Solid Edge part; units mm, degrees
sketch "Sketch1" plane through (0, 0, 0) normal (1, 0, 0) x (0, 1, 0)
  circle A0 centre (0, 0) radius 32
  circle A1 centre (0, 0) radius 16
extrude "Protrusion1" add sketch "Sketch1" against normal blind 70
sketch "Sketch2" plane through (0, 0, 0) normal (0, -1, 0) x (1, 0, 0)
  line L0 (-70, 32) -> (-36.8752, 123.9402)
  line L1 (0, 32) -> (0, 117.5)
  line L2 (0, 19.9591) -> (0, 32)
  line L3 (-70, 19.9591) -> (0, 19.9591)
  line L4 (-70, 32) -> (-70, 19.9591)
  arc A0 (-36.8752, 123.9402) -> (0, 117.5) centre (-19, 117.5) cw
extrude "ExtrudedProtrusion_6" add sketch "Sketch2" along normal mid plane 16
pattern_circular "Pattern1" count 3 over 360 about axis through (-70, 0, 0) along (-1, 0, 0) of "ExtrudedProtrusion_6"
sketch "Sketch3" plane through (0, 0, 25.9109) normal (1, 0, 0) x (0, -0.866, 0.5)
  line L0 (-29.1919, 50.0144) -> (-63.936, 110.2076)
  line L1 (-44.9554, 22.4395) -> (-114.4554, 22.4395)
  arc A0 (-114.4554, 22.4395) -> (-63.936, 110.2076) centre (-12.9554, 22.4395) cw
  arc A1 (-44.9554, 22.4395) -> (-29.1919, 50.0144) centre (-12.9554, 22.4395) cw
  circle A2 centre (-87.5005, 65.3234) radius 8
extrude "ExtrudedProtrusion_7" add sketch "Sketch3" against normal blind 19
pattern_circular "Pattern3" count 6 over 360 about axis through (0, 0, 0) along (-1, 0, 0) of "ExtrudedProtrusion_7"
sketch "Sketch4" plane through (-35, 76.5226, -34.9428) normal (0, 0.5, 0.866) x (0, 0.866, -0.5)
  circle A0 centre (33.7581, -16) radius 8
extrude "ExtrudedCutout_3" cut sketch "Sketch4" against normal blind 16
pattern_circular "Pattern4" count 3 over 360 about axis through (0, 0, 0) along (-1, 0, 0) of "ExtrudedCutout_3"
CAD build for the part. Positions are in the model's coordinates, mm. A direction names the side the tool comes from. Coordinates: 2 decimals unless noted, no trailing zeros. Order: outer loops, then holes, each group sorted by start corner. A loop starts at its lowest first (then second) coordinate and runs counter-clockwise, first axis right, second up. Notation, with made-up numbers: (-28.5, 24) - (10.5, 24) arc R17 cw to (10.5, 45) - close; hole circle Ø1 at (80, 12.25). An arc over 180 degrees is marked (long way). Use a Markdown table: item, result. Add a question column.
(1) Saw through at A-A (y = -55). Give the cut face in (x, z), then the cut area to 3 significant figures.
(2) Saw through at B-B (x = -54.5). Give the cut face in (y, z), then the cut area to 3 significant figures.
(3) Saw through at D-D (z = 0). Give the cut face in (x, y).
(4) Saw through at C-C (z = -36). Give the cut face in (x, y).
(5) Drill centre lines: line 1 along Y through (x, z) = (-14.5, 69); line 2 along Z through (x, y) = (-13.5, 79.5); line 3 along Y through (x, z) = (-32.5, -72). Where is each one in solid material? Low to high. Write a range as [from, to].
(6) Which spindle directions (+Z, -Z, +X, -X, +Y, -Y) get a long thin tool onto all of the face, cutting with end or side? Do faces 1 (the face through (-19, 38, 59)), 2 (the face through (-34.51, -57.73, -42.57)), 3 (the face through (-9.367, -57.52, 32.897)). Say none if no direction does.
(7) Pull direction Y, two halves, no side cores. Call faces 4 (the face through (-9.367, -57.386, 33.132)), 5 (the face through (0, -1, -18)), 6 (the face through (-53.67, 66.91, -38.76)), 7 (the face through (-9.367, -101.398, 4.556)): +Y half, -Y half, draft (parallel to the pull), parting line (faces both ways), or undercut.
(8) Flat gauge pins, fed straight in: pin 1 (3 mm diameter, centred on x = -15, z = 5, fed in from -Y); pin 2 (10 mm diameter, centred on x = -41, z = -24.5, fed in from +Y); pin 3 (9.5 mm diameter, centred on x = -12, z = -74, fed in from +Y); pin 4 (13 mm diameter, centred on y = 86, z = 0.13, fed in from -X). Where does each tip first touch, or does it go through?
Solved:
| question | item | result |
|---|---|---|
| 1 | outline | (-60.31, -22.52) - (-56.98, -40.99) - (-19, -40.99) - (-19, -85.31) - (0, -85.31) - (0, 31.44) - (-19, 31.44) - (-19, -22.52) - close; (-19, 31.75) - (0, 31.75) - (0, 85.31) - (-19, 85.31) - close |
| 1 | area | 3,970 mm² |
| 2 | outline | (-68.97, -30.58) - (-60.97, -44.44) - (-22.83, -22.42) arc R32 ccw to (22.83, -22.42) - (60.97, -44.44) - (68.97, -30.58) - (30.83, -8.56) arc R32 ccw to (8, 30.98) - (8, 75.02) - (-8, 75.02) - (-8, 30.98) arc R32 ccw to (-30.83, -8.56) - close; hole circle Ø32 at (0, 0) |
| 2 | area | 4,490 mm² |
| 3 | outline | (-70, -32) - (-19, -32) - (-19, -78) - (0, -78) - (0, -16) - (-70, -16) - close; (-70, 16) - (0, 16) - (0, 78) - (-19, 78) - (-19, 32) - (-70, 32) - close; (-19, -101.5) - (0, -101.5) - (0, -94) - (-19, -94) - close; (-19, 94) - (0, 94) - (0, 101.5) - (-19, 101.5) - close |
| 4 | outline | (-60.58, -46.35) - (-50.6, -78.35) - (-19, -78.35) - (-19, -94.9) - (0, -94.9) - (0, 0) - (-19, 0) - (-19, -46.35) - close; (-60.58, 46.35) - (-19, 46.35) - (-19, 0.27) - (0, 0.27) - (0, 94.9) - (-19, 94.9) - (-19, 78.35) - (-50.6, 78.35) - close |
| 5 | line 1 | y = [-74.44, -49.01], [-37.22, 37.12], [48.65, 74.44] |
| 5 | line 2 | z = [-63.1, -4.53], [4.8, 45.9], [46.21, 63.1] |
| 5 | line 3 | y = [-109.55, -108.71], [108.71, 109.55] |
| 6 | face 1 | +Z, -X, +Y |
| 6 | face 2 | -Z, -X |
| 6 | face 3 | +X, -X |
| 7 | face 4 | undercut |
| 7 | face 5 | draft |
| 7 | face 6 | +Y half |
| 7 | face 7 | -Y half |
| 8 | pin 1 | stops at y = -101.44 |
| 8 | pin 2 | stops at y = 67.1 |
| 8 | pin 3 | stops at y = 116.61 |
| 8 | pin 4 | passes through |
